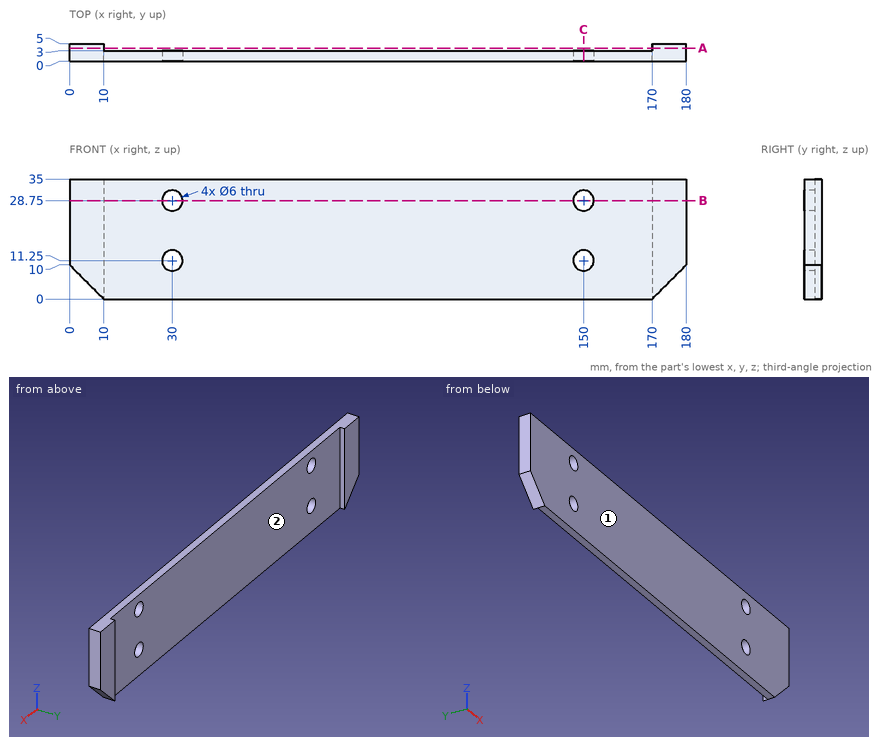
Geometry: see drawing. Coordinates: mm, zero at the bounding-box minimum. A direction names the side the tool comes from. Round coordinates to 2 decimals unless told otherwise and drop trailing zeros. Order: outer loops, then holes, each group sorted by start corner. A loop starts at its lowest first (then second) coordinate and runs counter-clockwise, first axis right, second up. Notation, with made-up numbers: (-39, 8.5) -> (-30, 8.5) arc R15 cw to (-30, 31.5) -> close; hole circle Ø7 at (37.25, -27.5). An arc over 180 degrees is marked (long way). Answer as CSV lines item,"result".
Item 1: Section A-A, the plane y = 3.8. Return loops of the section in (x, z).
A:
outline,"(0, 10) -> (10, 0) -> (10, 35) -> (0, 35) -> close; (170, 0) -> (180, 10) -> (180, 35) -> (170, 35) -> close"
Item 2: Section B-B, the plane z = 28.75. Return loops of the section in (x, y), plus the area to 3 significant figures.
A:
outline,"(0, 0) -> (27, 0) -> (27, 3) -> (10, 3) -> (10, 5) -> (0, 5) -> close; (33, 0) -> (147, 0) -> (147, 3) -> (33, 3) -> close; (153, 0) -> (180, 0) -> (180, 5) -> (170, 5) -> (170, 3) -> (153, 3) -> close"
area,"544 mm²"
Item 3: Line query: L1, parallel to Z at x = 150, y = 1.1; L2, parallel to X at y = 0.9, z = 11.25; L3, parallel to X at y = 4, z = 33. Output: solid intervals per line, ascending.
A:
L1,"0 to 8.25, 14.25 to 25.75, 31.75 to 35"
L2,"0 to 27, 33 to 147, 153 to 180"
L3,"0 to 10, 170 to 180"
Item 4: Section C-C, the plane x = 150. Return loops of the section in (y, z), plus the area to 3 significant figures.
A:
outline,"(0, 0) -> (3, 0) -> (3, 8.25) -> (0, 8.25) -> close; (0, 14.25) -> (3, 14.25) -> (3, 25.75) -> (0, 25.75) -> close; (0, 31.75) -> (3, 31.75) -> (3, 35) -> (0, 35) -> close"
area,"69.0 mm²"
Item 5: Pin query (flat end, axial travel): pin 1 Ø3.5 at (x, z) = (30, 28.75) entering from +Y; pin 2 Ø6 at (x, z) = (161, 10.5) entering from +Y. Return the tip coordinate at first contact, or that it passes through.
A:
pin 1,"through"
pin 2,"y = 3"
Item 6: Reachability of the marked faces 1 and 2 from +Z, -Z, +X, -X, +Y, -Y: full face, straight path, thin tool, end or side. Return the list, or none.
A:
face 1,"+Z, -Z, +X, -X, -Y"
face 2,"+Z, -Z, +Y"
